Design review of the part built by this model. Coordinates are the model's own, in mm. Face numbers are marked on the shaded views. A direction names the side the tool comes from. Round coordinates to 2 decimals unless told otherwise and drop trailing zeros. Order: outer loops, then holes, each group sorted by start corner. A loop starts at its lowest first (then second) coordinate and runs counter-clockwise, first axis right, second up. Notation, with made-up numbers: (22.5, 62) - (77.5, 62) arc R23 cw to (77.5, 88) - close; hole circle Ø9 at (-12.75, 77). An arc over 180 degrees is marked (long way). Write item = value, one per line.
from build123d import *

# Parameters (mm, degrees)
SKETCH1_W                     = 46.5
SKETCH1_H                     = 83
BOSS_EXTRUDE1_DEPTH           = 7.540625
CUT_EXTRUDE3_START            = 7.540625
CUT_EXTRUDE3_DEPTH            = 2.38125
SKETCH10_R                    = 1.35255
CUT_EXTRUDE6_DEPTH            = 4.76885
SKETCH11_W                    = 6.985
SKETCH11_H                    = 5.382155198
CUT_EXTRUDE7_DEPTH            = 2.38125
SKETCH12_R                    = 3.175
BOSS_EXTRUDE2_DEPTH           = 5.159375
BOSS_EXTRUDE2_DRAFT           = 1
BOSS_EXTRUDE2_PROFILE_2_DEPTH = 5.159375
BOSS_EXTRUDE2_PROFILE_2_DRAFT = 1
BOSS_EXTRUDE2_PROFILE_3_DEPTH = 5.159375
BOSS_EXTRUDE2_PROFILE_3_DRAFT = 1
SKETCH12_R_2                  = 2.38125
BOSS_EXTRUDE2_PROFILE_4_DEPTH = 5.159375
BOSS_EXTRUDE2_PROFILE_4_DRAFT = 1
FILLET1_R                     = 3.175
SKETCH13_R                    = 4.3053
CUT_EXTRUDE8_DEPTH            = 6.985
SKETCH14_R                    = 4.3053
CUT_EXTRUDE9_DEPTH            = 7.62


with BuildPart() as part:
    # Sketch1 → Boss-Extrude1 (new body)
    with BuildSketch(Plane(origin=(0, 0, 0), x_dir=(1, 0, 0), z_dir=(0, 1, 0))):
        Rectangle(SKETCH1_W, SKETCH1_H)
    extrude(amount=BOSS_EXTRUDE1_DEPTH)

    # Sketch2 → Cut-Extrude3 (cut)
    with BuildSketch(Plane(origin=(0, 0, 0), x_dir=(1, 0, 0), z_dir=(0, 1, 0)).offset(CUT_EXTRUDE3_START)):
        with BuildLine():
            Line((5.926342072, -15.8450122), (16.691855897, 34.802748287))
            ThreePointArc((16.691855897, 34.802748287), (16.847821053, 35.78747353), (16.9, 36.783107142))
            Line((16.9, 36.783107142), (16.9, 41.5))
            Line((16.9, 41.5), (10.55, 41.5))
            Line((10.55, 41.5), (10.55, 36.783107142))
            ThreePointArc((10.55, 36.783107142), (10.532607018, 36.451229271), (10.480618632, 36.122987524))
            Line((10.480618632, 36.122987524), (4.2, 6.575))
            Line((4.2, 6.575), (1.742353127, 18.137319476))
            ThreePointArc((1.742353127, 18.137319476), (-7.787687338, 36.612083158), (-13.035, 16.49730565))
            Line((-13.035, 16.49730565), (-13.035, -10.23))
            ThreePointArc((-13.035, -10.23), (-11.164876798, -14.744876798), (-6.65, -16.615))
            Line((-6.65, -16.615), (3.2078125, -16.615))
            Line((3.2078125, -16.615), (3.2078125, -20.512873774))
            ThreePointArc((3.2078125, -20.512873774), (2.656919843, -22.538622657), (1.155983232, -24.006386448))
            ThreePointArc((1.155983232, -24.006386448), (-2.044457088, -29.201835269), (0.7075, -34.648140337))
            Line((0.7075, -34.648140337), (0.7075, -41.5))
            Line((0.7075, -41.5), (7.6925, -41.5))
            Line((7.6925, -41.5), (7.6925, -34.648140337))
            ThreePointArc((7.6925, -34.648140337), (9.624653372, -32.569132052), (10.438131483, -29.8499878))
            Line((10.438131483, -29.8499878), (14.4748, -29.8499878))
            ThreePointArc((14.4748, -29.8499878), (17.575454609, -28.565654609), (18.8597878, -25.465))
            Line((18.8597878, -25.465), (18.8597878, -20.23))
            ThreePointArc((18.8597878, -20.23), (17.575454609, -17.129345391), (14.4748, -15.8450122))
            Line((14.4748, -15.8450122), (5.926342072, -15.8450122))
        make_face()
        with BuildLine():
            Line((14.4748, -29.08), (10.43813073, -29.08))
            ThreePointArc((10.43813073, -29.08), (9.489135484, -26.135203334), (7.244016768, -24.006386448))
            ThreePointArc((7.244016768, -24.006386448), (5.743080157, -22.538622657), (5.1921875, -20.512873774))
            Line((5.1921875, -20.512873774), (5.1921875, -16.615))
            Line((5.1921875, -16.615), (14.4748, -16.615))
            ThreePointArc((14.4748, -16.615), (17.030991014, -17.673808986), (18.0898, -20.23))
            Line((18.0898, -20.23), (18.0898, -25.465))
            ThreePointArc((18.0898, -25.465), (17.030991014, -28.021191014), (14.4748, -29.08))
        make_face(mode=Mode.SUBTRACT)
        with BuildLine():
            Line((-4.021712531, 14.713303237), (2.473657928, -15.8450122))
            Line((2.473657928, -15.8450122), (-6.65, -15.8450122))
            ThreePointArc((-6.65, -15.8450122), (-10.620413203, -14.200413203), (-12.2650122, -10.23))
            Line((-12.2650122, -10.23), (-12.2650122, 15.993340762))
            ThreePointArc((-12.2650122, 15.993340762), (-8.267823292, 14.551807439), (-4.021712531, 14.713303237))
        make_face(mode=Mode.SUBTRACT)
    extrude(amount=-CUT_EXTRUDE3_DEPTH, mode=Mode.SUBTRACT)

    # Sketch10 → Cut-Extrude6 (cut)
    with BuildSketch(Plane(origin=(0, 7.540625, 0), x_dir=(1, 0, 0), z_dir=(0, 1, 0))):
        with Locations(Location((18.4747939, -22.8475, 0), (0, 0, 270))):
            Circle(SKETCH10_R)
        with Locations(Location((-12.6500061, 3.133652825, 0), (0, 0, 270))):
            Circle(SKETCH10_R)
    extrude(amount=-CUT_EXTRUDE6_DEPTH, mode=Mode.SUBTRACT)

    # Sketch11 → Cut-Extrude7 (cut)
    with BuildSketch(Plane(origin=(0, 7.540625, 0), x_dir=(1, 0, 0), z_dir=(0, 1, 0))):
        with Locations((-6.56, 38.808922401)):
            Rectangle(SKETCH11_W, SKETCH11_H)
    extrude(amount=-CUT_EXTRUDE7_DEPTH, mode=Mode.SUBTRACT)


with BuildPart() as boss_extrude2_tool:
    # Sketch12 → Boss-Extrude2 (with draft: the straight prism first)
    with BuildSketch(Plane(origin=(0, 7.540625, 0), x_dir=(1, 0, 0), z_dir=(0, 1, 0))):
        with Locations((-16.9, -35.15)):
            Circle(SKETCH12_R)
    extrude(amount=BOSS_EXTRUDE2_DEPTH)
    # Boss-Extrude2: the draft: its side faces are tilted about the plane it starts from
    boss_extrude2_sides = [boss_extrude2_tool.faces().sort_by_distance(p)[0] for p in [
        (-20.075, 10.1203125, 35.15),
    ]]
    draft(boss_extrude2_sides, Plane(origin=(0, 7.540625, 0), x_dir=(1, 0, 0), z_dir=(0, 1, 0)), BOSS_EXTRUDE2_DRAFT)


with BuildPart() as part_1:
    add(part.part)

    # Boss-Extrude2: add boss_extrude2_tool
    add(boss_extrude2_tool.part)


with BuildPart() as boss_extrude2_profile_2_tool:
    # Sketch12 → Boss-Extrude2 profile 2 (with draft: the straight prism first)
    with BuildSketch(Plane(origin=(0, 7.540625, 0), x_dir=(1, 0, 0), z_dir=(0, 1, 0))):
        with Locations((16.9, -35.15)):
            Circle(SKETCH12_R)
    extrude(amount=BOSS_EXTRUDE2_PROFILE_2_DEPTH)
    # Boss-Extrude2 profile 2: the draft: its side faces are tilted about the plane it starts from
    boss_extrude2_profile_2_sides = [boss_extrude2_profile_2_tool.faces().sort_by_distance(p)[0] for p in [
        (13.725, 10.1203125, 35.15),
    ]]
    draft(boss_extrude2_profile_2_sides, Plane(origin=(0, 7.540625, 0), x_dir=(1, 0, 0), z_dir=(0, 1, 0)), BOSS_EXTRUDE2_PROFILE_2_DRAFT)


with BuildPart() as part_2:
    add(part_1.part)

    # Boss-Extrude2 profile 2: add boss_extrude2_profile_2_tool
    add(boss_extrude2_profile_2_tool.part)


with BuildPart() as boss_extrude2_profile_3_tool:
    # Sketch12 → Boss-Extrude2 profile 3 (with draft: the straight prism first)
    with BuildSketch(Plane(origin=(0, 7.540625, 0), x_dir=(1, 0, 0), z_dir=(0, 1, 0))):
        with Locations((16.9, 9.75)):
            Circle(SKETCH12_R)
    extrude(amount=BOSS_EXTRUDE2_PROFILE_3_DEPTH)
    # Boss-Extrude2 profile 3: the draft: its side faces are tilted about the plane it starts from
    boss_extrude2_profile_3_sides = [boss_extrude2_profile_3_tool.faces().sort_by_distance(p)[0] for p in [
        (13.725, 10.1203125, -9.75),
    ]]
    draft(boss_extrude2_profile_3_sides, Plane(origin=(0, 7.540625, 0), x_dir=(1, 0, 0), z_dir=(0, 1, 0)), BOSS_EXTRUDE2_PROFILE_3_DRAFT)


with BuildPart() as part_3:
    add(part_2.part)

    # Boss-Extrude2 profile 3: add boss_extrude2_profile_3_tool
    add(boss_extrude2_profile_3_tool.part)


with BuildPart() as boss_extrude2_profile_4_tool:
    # Sketch12 → Boss-Extrude2 profile 4 (with draft: the straight prism first)
    with BuildSketch(Plane(origin=(0, 7.540625, 0), x_dir=(1, 0, 0), z_dir=(0, 1, 0))):
        with Locations((-18.4748, 36.7375)):
            Circle(SKETCH12_R_2)
    extrude(amount=BOSS_EXTRUDE2_PROFILE_4_DEPTH)
    # Boss-Extrude2 profile 4: the draft: its side faces are tilted about the plane it starts from
    boss_extrude2_profile_4_sides = [boss_extrude2_profile_4_tool.faces().sort_by_distance(p)[0] for p in [
        (-20.85605, 10.1203125, -36.7375),
    ]]
    draft(boss_extrude2_profile_4_sides, Plane(origin=(0, 7.540625, 0), x_dir=(1, 0, 0), z_dir=(0, 1, 0)), BOSS_EXTRUDE2_PROFILE_4_DRAFT)


with BuildPart() as part_4:
    add(part_3.part)

    # Boss-Extrude2 profile 4: add boss_extrude2_profile_4_tool
    add(boss_extrude2_profile_4_tool.part)

    # Fillet1
    fillet1_edges = [part_4.edges().sort_by_distance(p)[0] for p in [
        (23.25, 3.7703125, 41.5),
        (-23.25, 3.7703125, 41.5),
        (-23.25, 3.7703125, -41.5),
    ]]
    fillet(fillet1_edges, radius=FILLET1_R)

    # Sketch13 → Cut-Extrude8 (cut)
    with BuildSketch(Plane(origin=(0, 0, -41.5), x_dir=(-1, 0, 0), z_dir=(0, 0, -1))):
        with Locations((-13.725, 6.35)):
            Circle(SKETCH13_R)
        with Locations((6.56, 6.35)):
            Circle(SKETCH13_R)
    extrude(amount=-CUT_EXTRUDE8_DEPTH, mode=Mode.SUBTRACT)

    # Sketch14 → Cut-Extrude9 (cut)
    with BuildSketch(Plane.XY.offset(41.5)):
        with Locations((4.2, 6.35)):
            Circle(SKETCH14_R)
    extrude(amount=-CUT_EXTRUDE9_DEPTH, mode=Mode.SUBTRACT)


solid = part_4.part
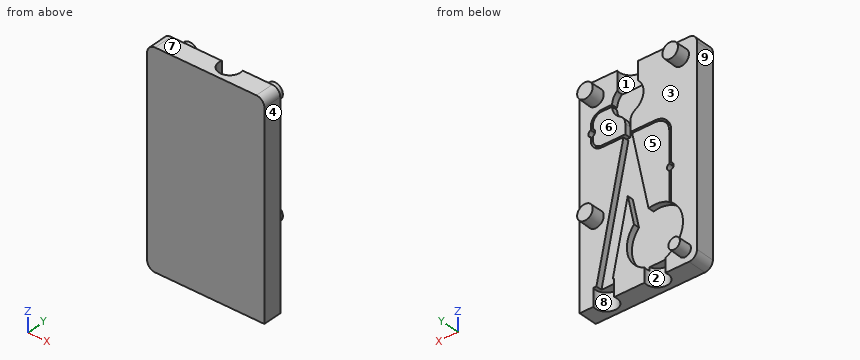
Item 1: Insertion check: P1, Ø2, axis at x = 19, z = 23, coming from the +Y side; P2, Ø1.5, axis at x = -17, y = 9, coming from the -Z side; P3, Ø2.5, axis at x = -7, y = 3.5, coming from the -Z side (3 decimals). Each pin has a flat end and moves straight along its axis. Give the tip position at first contact, or say it passes through.
Data:
P1 = 7.54
P2 = -38.98
P3 = -34.515
Item 2: Take a section at C-C, the plane z = -1. State the section outline as (x, y) points (3 decimals).
Data:
outline = (-23.25, 0) - (23.25, 0) - (23.25, 7.541) - (9.507, 7.541) - (9.507, 5.159) - (-1.107, 5.159) - (-1.107, 7.541) - (-12.265, 7.541) - (-12.265, 5.159) - (-13.035, 5.159) - (-13.035, 7.541) - (-23.25, 7.541) - close
Item 3: Take a section at D-D, the plane y = 11. State the section outline as (x, z) points.
Data:
outline = circle Ø4.64 at (-18.47, -36.74); circle Ø6.23 at (-16.9, 35.15); circle Ø6.23 at (16.9, -9.75); circle Ø6.23 at (16.9, 35.15)
Item 4: For the marked faces 5, 6, 7, 8 and 9, list the 3-axis set-ups (+Z, -Z, +X, -X, +Y, -Y) from which the entire face can be reached by the end or side of a thin tool; tool diameter is ignored.
Data:
face_5 = +Z, -Z, -X, +Y
face_6 = +X, -X, +Y
face_7 = +Z, +X, -X, +Y, -Y
face_8 = -Z
face_9 = +Z, -Z, -X, +Y, -Y
Item 5: Take a section at A-A, the plane x = 12. State the section outline as (y, z) points (3 decimals).
Data:
outline = (0, -41.5) - (2.405, -41.5) - (2.405, -34.515) - (5.159, -34.515) - (5.159, -12.729) - (7.541, -12.729) - (7.541, 15.845) - (5.159, 15.845) - (5.159, 16.615) - (7.541, 16.615) - (7.541, 29.08) - (5.159, 29.08) - (5.159, 29.85) - (7.541, 29.85) - (7.541, 41.5) - (0, 41.5) - close
Item 6: The part is to be moulded in two halves that separate along Y. For the marked faces 1, 2, 3 and 4, say which applies: +Y half, -Y half, draft (parallel to the pull), parting line (faces both ways), or undercut.
Data:
face_1 = undercut
face_2 = undercut
face_3 = +Y half
face_4 = draft
Item 7: For line 1 along X through (y, z) = (6.35, 36.25); line 2 along X through (y, z) = (7, -34); line 3 along Y through (x, z) = (-6.56, -37), list the stretches that pass through material, from the lowest coordinate up. Write a range as [from, to].
Data:
line_1 = [-23.25, -0.11], [8.51, 23.25]
line_2 = [-23.25, -13.8], [0.68, 10.03], [16.52, 23.25]
line_3 = [0, 2.04]
Item 8: Take a section at B-B, the plane y = 3.75. Count the separate pieces of the cut face and the enclosed holes in it, and give its area (3 significant figures).
Data:
separate_pieces = 1
enclosed_holes = 2
area = 3,690 mm2
